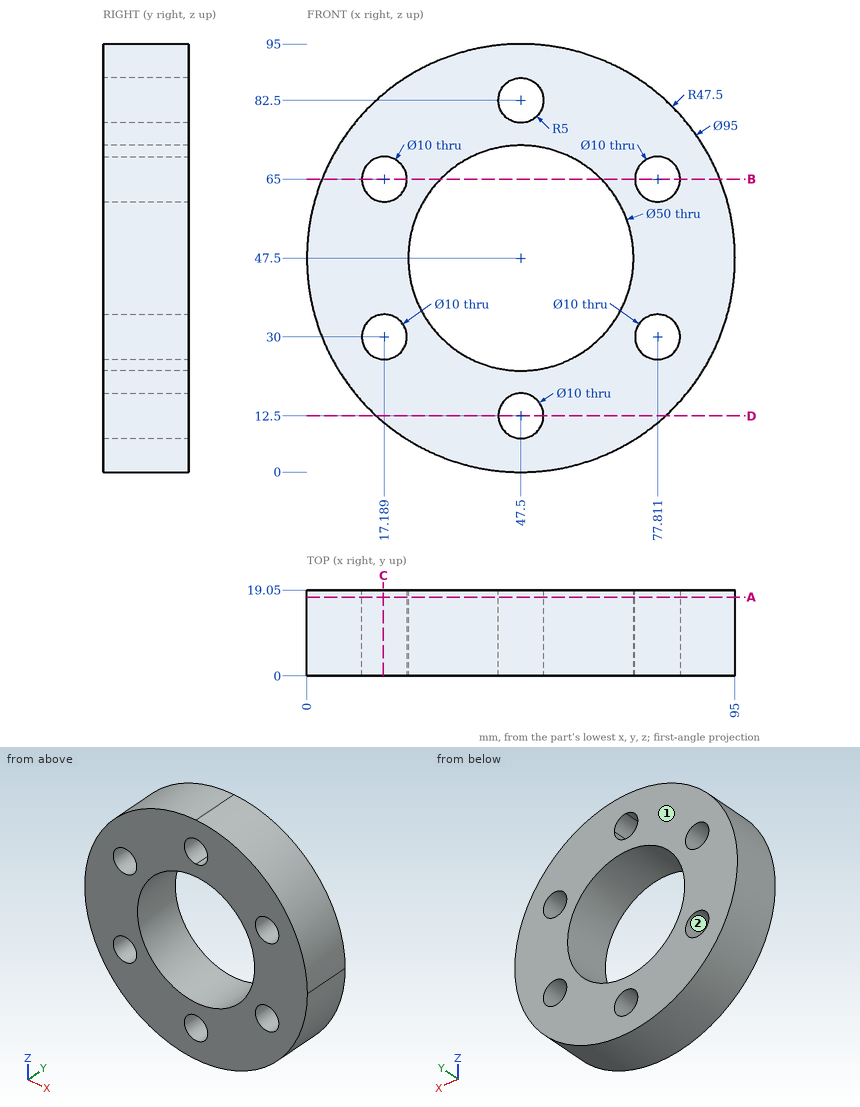
Verification items for this drawing (mm, ordinates from the low corner). Give positions to 0.01 mm unless a question says otherwise; leave off trailing zeros. Write each loop counter-clockwise with the first axis right and the second up, starting at its lowest first coordinate (ties: lowest second). Pieces come first, ordered by that corner, then holes.
1) Cross-section at D-D (z = 12.5). Record the boundary of the cut face in (x, y), plus the area to 3 significant figures.
Values follow:
outline: (15.39, 0) - (42.5, 0) - (42.5, 19.05) - (15.39, 19.05) - close; (52.5, 0) - (79.61, 0) - (79.61, 19.05) - (52.5, 19.05) - close
area: 1,030 mm2
2) Cross-section at C-C (x = 17). Record the boundary of the cut face in (y, z), plus the area to 3 significant figures.
Values follow:
outline: (0, 11.09) - (19.05, 11.09) - (19.05, 25) - (0, 25) - close; (0, 35) - (19.05, 35) - (19.05, 60) - (0, 60) - close; (0, 70) - (19.05, 70) - (19.05, 83.91) - (0, 83.91) - close
area: 1,010 mm2
3) Go/stop test with flat-tipped pins: pin 1 Ø6 at (y, z) = (5.5, 22.5) entering from -X; pin 2 Ø8 at (x, z) = (17.19, 30) entering from +Y; pin 3 Ø1 at (x, y) = (43.5, 4) entering from +Z; pin 4 Ø5 at (y, z) = (6.5, 69) entering from +X. Record where each tip stops, or that it passes through.
Values follow:
pin 1: stops at x = 5.4
pin 2: passes through
pin 3: stops at z = 94.87
pin 4: stops at x = 91.03
4) Thickness scan on line 1 (X direction, y = 5.5, z = 69) (1 decimal); line 2 (Z direction, x = 51, y = 11.5); line 3 (Z direction, x = 76.5, y = 7.5) (1 decimal). Record the ranges inside material, lowest first.
Values follow:
line 1: x = 5.1 to 14.2, 20.2 to 34.7, 60.3 to 74.8, 80.8 to 89.9
line 2: z = 0.13 to 8.93, 16.07 to 22.75, 72.25 to 78.93, 86.07 to 94.87
line 3: z = 9.9 to 25.2, 34.8 to 60.2, 69.8 to 85.1
5) Cross-section at A-A (y = 17.5). Record the boundary of the cut face in (x, z).
Values follow:
outline: circle Ø95 at (47.5, 47.5); hole circle Ø10 at (17.19, 30); hole circle Ø10 at (17.19, 65); hole circle Ø50 at (47.5, 47.5); hole circle Ø10 at (47.5, 12.5); hole circle Ø10 at (47.5, 82.5); hole circle Ø10 at (77.81, 30); hole circle Ø10 at (77.81, 65)
6) Cross-section at B-B (z = 65). Record the boundary of the cut face in (x, y).
Values follow:
outline: (3.34, 0) - (12.19, 0) - (12.19, 19.05) - (3.34, 19.05) - close; (22.19, 0) - (29.65, 0) - (29.65, 19.05) - (22.19, 19.05) - close; (65.35, 0) - (72.81, 0) - (72.81, 19.05) - (65.35, 19.05) - close; (82.81, 0) - (91.66, 0) - (91.66, 19.05) - (82.81, 19.05) - close
7) Release check for a two-part mould opening along Z. For the marked faces 1 and 2 record: released by +Z, released by -Z, zero draft, split by the parting line, or undercut.
Values follow:
face 1: zero draft
face 2: undercut
